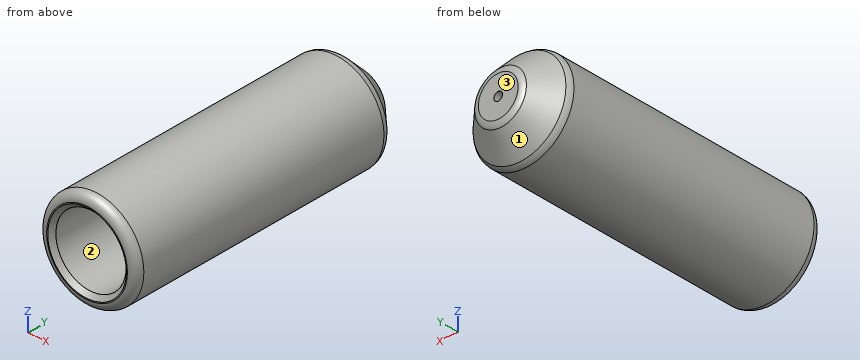
```python
from build123d import *

# Parameters (mm, degrees)
CHAMFER1_SIZE = 3
FILLET1_R     = 1
CHAMFER2_SIZE = 0.5


with BuildPart() as part:
    # Sketch1 → Revolve1 (revolve)
    with BuildSketch(Plane.XY):
        with BuildLine():
            Line((5.75, 0), (5.75, 35))
            Line((5.75, 35), (0.5, 35))
            Line((0.5, 35), (0.5, 33.414213562))
            ThreePointArc((0.5, 33.414213562), (0.576120467, 33.03153013), (0.792893219, 32.707106781))
            Line((0.792893219, 32.707106781), (1.707106781, 31.792893219))
            ThreePointArc((1.707106781, 31.792893219), (1.923879533, 31.46846987), (2, 31.085786438))
            Line((2, 31.085786438), (2, 26))
            ThreePointArc((2, 26), (2.292893219, 25.292893219), (3, 25))
            Line((3, 25), (3.125, 25))
            ThreePointArc((3.125, 25), (3.832106781, 24.707106781), (4.125, 24))
            Line((4.125, 24), (4.125, 0))
            Line((4.125, 0), (5.75, 0))
        make_face()
    revolve(axis=Axis((0, -1000, 0), (0, 1, 0)))

    # Chamfer1
    chamfer1_edges = [part.edges().sort_by_distance(p)[0] for p in [
        (-5.75, 35, 0),
    ]]
    chamfer(chamfer1_edges, length=CHAMFER1_SIZE)

    # Fillet1
    fillet1_edges = [part.edges().sort_by_distance(p)[0] for p in [
        (-5.75, 0, 0),
        (-5.75, 32, 0),
        (-2.75, 35, 0),
    ]]
    fillet(fillet1_edges, radius=FILLET1_R)

    # Chamfer2
    chamfer2_edges = [part.edges().sort_by_distance(p)[0] for p in [
        (-4.125, 0, 0),
    ]]
    chamfer(chamfer2_edges, length=CHAMFER2_SIZE)


solid = part.part
```
For this review, take the finished solid that the model builds, in its own axes (mm). Face numbers are marked on the shaded views. Round coordinates to 2 decimals unless told otherwise and drop trailing zeros. Write each loop counter-clockwise with the first axis right and the second up, starting at its lowest first coordinate (ties: lowest second). Pieces come first, ordered by that corner, then holes. Notation, with made-up numbers: (7.25, 18) -> (47.25, 18) arc R14 ccw to (47.25, 22) -> close; hole circle Ø4 at (69.5, -21). An arc over 180 degrees is marked (long way). One line per question, with ' | ' between items. Start each with the question number.
1) Add section A-A (y = 8). Write out the cut boundary in (x, z) (3 decimals).
2) Wall thickness on line 1 along X through (y, z) = (27.75, 0); line 2 along X through (y, z) = (7.25, 0) (3 decimals): over which ranges is each line inside the solid? List them lowest first.
3) For pin 1 Ø1.5 at (x, y) = (-2, 5.5) entering from -Z; pin 2 Ø6 at (x, y) = (-4, 11.5) entering from -Z; pin 3 Ø6.5 at (x, z) = (0, 0) entering from -Y; pin 4 Ø6.5 at (x, z) = (0, 0) entering from +Y, all flat-tipped, find the tip position at first contact; note any pin that passes through.
4) Add section B-B (y = 24.5). Write out the cut boundary in (x, z).
5) Mouldability with a two-part tool opening along X and no side actions: class the marked faces 1, 2 and 3 as +X half, -X half, draft (parallel to the pull), parting line (faces both ways), or undercut.
Reported:
1) outline: circle Ø11.5 at (0, 0); hole circle Ø8.25 at (0, 0)
2) line 1: x = -5.75 to -2, 2 to 5.75 | line 2: x = -5.75 to -4.125, 4.125 to 5.75
3) pin 1: stops at z = -5.61 | pin 2: stops at z = -5.66 | pin 3: stops at y = 24.99 | pin 4: stops at y = 35
4) outline: circle Ø11.5 at (0, 0); hole circle Ø7.98 at (0, 0)
5) face 1: parting line | face 2: undercut | face 3: draft
